Source: CAD feature listing. Evaluate the final solid. Frame: model axes, mm. Face numbers are marked on the shaded views. A direction names the side the tool comes from. Give positions to 0.01 mm unless a question says otherwise; leave off trailing zeros. Loops run counter-clockwise (first coordinate to the right, second up) from the corner with the lowest first, then second, coordinate; pieces in that order, holes last. Notation, with made-up numbers: (42.25, -19.5) -> (83.25, -19.5) arc R30 ccw to (83.25, 3.5) -> close; hole circle Ø5 at (76.25, -4). An arc over 180 degrees is marked (long way). Put each result on its own line as item: value.
```python
from build123d import *

# Parameters (mm, degrees)
CIRPATTERN_COUNT = 8
SLOT_CUT_DEPTH   = 196.79823157


with BuildPart() as part:
    # Sketch1 → Revolve 2 (revolve)
    with BuildSketch(Plane.XY, mode=Mode.PRIVATE) as revolve_2_sk:
        Polygon((0, 43.897637795), (30, 43.897637795), (75, -1.102362205), (75, -56.102362205), (63, -56.102362205), (63, -6.072924953), (25.029437252, 31.897637795), (0, 31.897637795), align=None)
    revolve(revolve_2_sk.sketch.rotate(Axis((63, -56.102362205, 0), (1, 0, 0)), 90), axis=Axis((63, -56.102362205, 0), (1, 0, 0)))

    # Sketch3 → M8x1.0 Tapped Hole (revolve, cut)
    with BuildSketch(Plane.ZX.offset(37.897637795)):
        Polygon((0, 0), (0, 23.103012167), (3.5, 21), (3.5, 0), align=None)
    m8x1_0_tapped_hole = revolve(axis=Axis((-6.35, 37.897637795, 0), (1, 0, 0)), mode=Mode.SUBTRACT)

    # CirPattern: M8x1.0 Tapped Hole ×8 about axis
    cirpattern_axis = Axis((0, -56.102362205, 0), (1, 0, 0))
    for i in range(1, CIRPATTERN_COUNT):
        add(m8x1_0_tapped_hole.rotate(cirpattern_axis, i * 360 / CIRPATTERN_COUNT), mode=Mode.SUBTRACT)

    # Sketch2 → Slot Cut (cut, through all)
    with BuildSketch(Plane.ZY.offset(-63)):
        with BuildLine():
            Line((-15, -37.602362205), (15, -37.602362205))
            ThreePointArc((15, -37.602362205), (21, -43.602362205), (15, -49.602362205))
            Line((15, -49.602362205), (-15, -49.602362205))
            ThreePointArc((-15, -49.602362205), (-21, -43.602362205), (-15, -37.602362205))
        make_face()
    slot_cut = extrude(amount=-SLOT_CUT_DEPTH, mode=Mode.SUBTRACT)

    # Mirror 2: Slot Cut across plane
    add(slot_cut.mirror(Plane.ZX.offset(-56.102362205)), mode=Mode.SUBTRACT)


solid = part.part
```
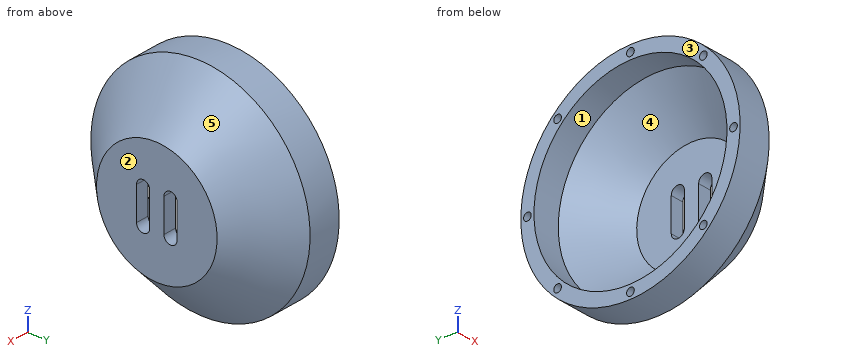
(1) Section A-A on x = 18. Give the number of separate pieces and of enclosed holes in the cut face, then the cut area to 3 significant figures.
Calculated:
separate pieces: 1
enclosed holes: 9
area: 6,780 mm²
(2) Reachability of the marked faces 1 and 2 from +Z, -Z, +X, -X, +Y, -Y: full face, straight path, thin tool, end or side. Return the list, or none.
Calculated:
face 1: -X
face 2: +Z, -Z, +X, +Y, -Y
(3) Draft query along Y for the marked faces 3, 4 and 5. Return one class per face: released by +Y, released by -Y, zero draft, split by the parting line, or undercut.
Calculated:
face 3: zero draft
face 4: undercut
face 5: split by the parting line
(4) Section B-B on x = 47.5. Return loops of the section in (y, z).
Calculated:
outline: circle Ø165 at (-56.1, 0); hole circle Ø131.06 at (-56.1, 0)
(5) Line query: probe 1 along Y at (x, z) = (9.75, 0); probe 2 along Z at (x, y) = (16, 7.5); probe 3 along Y at (x, z) = (11, 68.5) (3 decimals). Output: solid intervals per line, ascending. Write a range as from..to.
Calculated:
probe 1: y = -156.1..-153.6, -146.6..-144.1, 31.9..34.4, 41.4..43.9
probe 2: z = -77.17..-68.48, -64.46..-60.82, 60.82..64.46, 68.48..77.17
probe 3: y = -128.957..-125.42, -119.721..-111.345, -0.86..7.516, 13.215..16.752
(6) First-contact query: P1, Ø1.5, axis at x = 37, z = -1, coming from the -Y side; P2, Ø8, axis at x = 56.5, y = 9.5, coming from the +Z side; P3, Ø6, axis at x = 72, z = 1.5, coming from the -Y side. Flat tips, straight axial feed; report the tip coordinate or a pass-through.
Calculated:
P1: stops at y = -149.85
P2: stops at z = 43.46
P3: stops at y = -117.08
